The model under review builds one solid part; all positions refer to its coordinate system, in mm. Round coordinates to 2 decimals unless told otherwise and drop trailing zeros. Order: outer loops, then holes, each group sorted by start corner. A loop starts at its lowest first (then second) coordinate and runs counter-clockwise, first axis right, second up. Notation, with made-up numbers: (21.5, 32) -> (28.5, 32) arc R16 ccw to (28.5, 55) -> close; hole circle Ø8 at (49.25, 46). An arc over 180 degrees is marked (long way). Use a Markdown table: item, result. Add a question column.
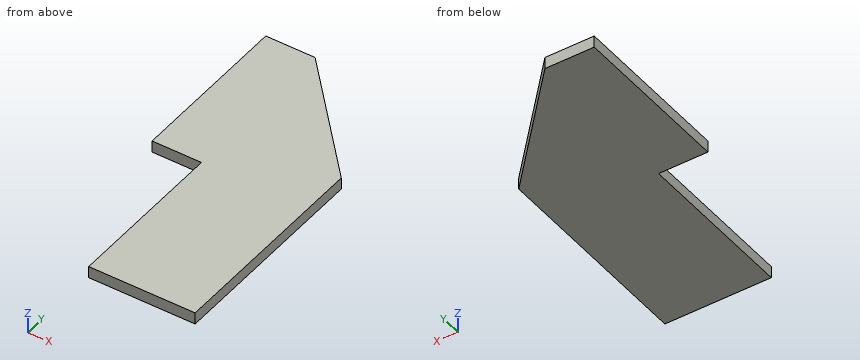
Autodesk Inventor part; units mm, degrees
ref_plane "YZ Plane" through (0, 0, 0) normal (1, 0, 0) x (0, 1, 0)
ref_plane "XZ Plane" through (0, 0, 0) normal (0, 1, 0) x (-1, 0, 0)
ref_plane "XY Plane" through (0, 0, 0) normal (0, 0, 1) x (1, 0, 0)
sketch "Sketch1" plane through (0, 0, 0) normal (0, 0, 1) x (1, 0, 0)
  line L0 (0, 0) -> (114.3, 0)
  line L1 (114.3, 0) -> (114.3, 228.6)
  line L2 (114.3, 228.6) -> (0, 228.6)
  line L3 (0, 228.6) -> (0, 0)
  dimension "d0" = 114.3
  dimension "d1" = 228.6
extrude "Extrusion1" add sketch "Sketch1" along normal blind 12.7
sketch "Sketch3" plane through (0, 0, 12.7) normal (0, 0, 1) x (1, 0, 0)
  line L0 (114.3, 0) -> (114.3, 228.6)
  line L1 (114.3, 228.6) -> (0, 354.1146)
  line L2 (0, 354.1146) -> (0, 228.6)
  line L3 (0, 228.6) -> (114.3, 228.6)
  point P0 (0, 0)
extrude "Extrusion2" add sketch "Sketch3" against normal blind 12.7
sketch "Sketch4" plane through (0, 0, 0) normal (0, 0, -1) x (-1, 0, 0)
  line L0 (0, 354.1146) -> (52.993, 354.1146)
  line L1 (52.993, 354.1146) -> (52.993, 176.3146)
  line L2 (52.993, 176.3146) -> (0, 176.3146)
  line L3 (0, 176.3146) -> (0, 354.1146)
  point P0 (0, 0)
  point P1 (0, 354.1146)
  dimension "d7" = 177.8
extrude "Extrusion3" add sketch "Sketch4" against normal blind 12.7
properties part number "motor mount platform"
Q1. Add section C-C (x = -8). Write out the cut boundary in (y, z), then the cut area to 3 significant figures.
Q2. Add section B-B (y = 108). Write out the cut boundary in (x, z), then the cut area to 3 significant figures.
Q3. Insertion check: pin 1 (4 mm diameter, centred on y = 90.5, z = 8, fed in from -X); pin 2 (3 mm diameter, centred on x = 70.5, z = 10.5, fed in from -Y); pin 3 (1 mm diameter, centred on x = 20.5, z = 8.5, fed in from +Y). Each pin has a flat end and moves straight along its axis. Give the tip position at first contact, or say it passes through.
Q4. Add section A-A (z = 10.25). Write out the cut boundary in (x, y).
Q5. Wall thickness on line 1 (Y direction, x = -1.5, z = 7.5); line 2 (X direction, y = 156, z = 12.25); line 3 (Y direction, x = 13, z = 7.5): over which ranges is each line inside the solid? List them lowest first. Write a range as [from, to].
Report:
| question | item | result |
|---|---|---|
| 1 | outline | (176.31, 0) -> (354.11, 0) -> (354.11, 12.7) -> (176.31, 12.7) -> close |
| 1 | area | 2,260 mm² |
| 2 | outline | (0, 0) -> (114.3, 0) -> (114.3, 12.7) -> (0, 12.7) -> close |
| 2 | area | 1,450 mm² |
| 3 | pin 1 | stops at x = 0 |
| 3 | pin 2 | stops at y = 0 |
| 3 | pin 3 | stops at y = 332.15 |
| 4 | outline | (-52.99, 176.31) -> (0, 176.31) -> (0, 0) -> (114.3, 0) -> (114.3, 228.6) -> (0, 354.11) -> (-52.99, 354.11) -> close |
| 5 | line 1 | y = [176.31, 354.11] |
| 5 | line 2 | x = [0, 114.3] |
| 5 | line 3 | y = [0, 339.84] |
